```python
from build123d import *

# Parameters (mm, degrees)
SKETCH1_W            = 254
SKETCH1_H            = 203.2
BOSS_EXTRUDE2_DEPTH  = 12.7
SKETCH2_W            = 254
SKETCH2_H            = 203.2
SKETCH2_W_2          = 228.6
SKETCH2_H_2          = 177.8
BOSS_EXTRUDE3_DEPTH  = 12.7
SKETCH6_R            = 6.35
CUT_EXTRUDE2_DEPTH   = 52.07
SKETCH8_R            = 6.35
CUT_EXTRUDE3_DEPTH   = 52.07
SKETCH9_R            = 3.302
BOSS_EXTRUDE5_DEPTH  = 25.4
SKETCH10_R           = 6.35
CUT_EXTRUDE4_DEPTH   = 45.212
SKETCH11_R           = 6.35
CUT_EXTRUDE5_DEPTH   = 190.246
SKETCH12_R           = 5.842
SKETCH12_R_2         = 3.302
BOSS_EXTRUDE6_DEPTH  = 24.13
SKETCH15_R           = 6.35
CUT_EXTRUDE6_DEPTH   = 1.27
SKETCH17_R           = 3.302
BOSS_EXTRUDE7_DEPTH  = 1.27
SKETCH18_R           = 3.302
BOSS_EXTRUDE8_DEPTH  = 1.27
SKETCH19_R           = 5.842
SKETCH19_R_2         = 3.302
BOSS_EXTRUDE9_DEPTH  = 73.025
CUT_EXTRUDE7_DEPTH   = 7.62
SKETCH21_R           = 6.35
BOSS_EXTRUDE10_DEPTH = 12.7
SKETCH23_R           = 6.35
BOSS_EXTRUDE11_DEPTH = 12.7
SKETCH24_R           = 3.81
CUT_EXTRUDE8_DEPTH   = 167.132
FILLET1_R            = 5.08


with BuildPart() as part:
    # Sketch1 → Boss-Extrude2 (new body)
    with BuildSketch(Plane(origin=(0, 0, 0), x_dir=(1, 0, 0), z_dir=(0, 1, 0))):
        with Locations((127, 101.6)):
            Rectangle(SKETCH1_W, SKETCH1_H)
    extrude(amount=BOSS_EXTRUDE2_DEPTH)

    # Sketch2 → Boss-Extrude3 (add)
    with BuildSketch(Plane(origin=(0, 0, 0), x_dir=(-1, 0, 0), z_dir=(0, -1, 0))):
        with Locations((-127, 101.6)):
            Rectangle(SKETCH2_W, SKETCH2_H)
        with Locations((-127, 101.6)):
            Rectangle(SKETCH2_W_2, SKETCH2_H_2, mode=Mode.SUBTRACT)
    extrude(amount=BOSS_EXTRUDE3_DEPTH)

    # Sketch6 → Cut-Extrude2 (cut)
    with BuildSketch(Plane(origin=(228.6, 0, 0), x_dir=(0, 0, -1), z_dir=(1, 0, 0))):
        with Locations((0, -12.7)):
            Circle(SKETCH6_R)
    extrude(amount=-CUT_EXTRUDE2_DEPTH, mode=Mode.SUBTRACT)

    # Sketch8 → Cut-Extrude3 (cut)
    with BuildSketch(Plane.ZY.offset(-25.4)):
        with Locations((0, -12.7)):
            Circle(SKETCH8_R)
    extrude(amount=-CUT_EXTRUDE3_DEPTH, mode=Mode.SUBTRACT)

    # Sketch9 → Boss-Extrude5 (add)
    with BuildSketch(Plane(origin=(228.6, 0, 0), x_dir=(0, 0, -1), z_dir=(1, 0, 0))):
        with BuildLine():
            Line((0, -4.734153711), (0, -6.858))
            ThreePointArc((0, -6.858), (-4.130917816, -16.830917816), (5.842, -12.7))
            Line((5.842, -12.7), (6.842694324, -12.7))
            Line((6.842694324, -12.7), (6.842694324, -8.927228158))
            Line((6.842694324, -8.927228158), (0, -4.734153711))
        make_face()
        with Locations((0, -12.7)):
            Circle(SKETCH9_R, mode=Mode.SUBTRACT)
    extrude(amount=-BOSS_EXTRUDE5_DEPTH)

    # Sketch10 → Cut-Extrude4 (cut)
    with BuildSketch(Plane(origin=(228.6, 0, 0), x_dir=(0, 0, -1), z_dir=(1, 0, 0))):
        with Locations((0, -12.7)):
            Circle(SKETCH10_R)
    extrude(amount=CUT_EXTRUDE4_DEPTH, mode=Mode.SUBTRACT)

    # Sketch11 → Cut-Extrude5 (cut)
    with BuildSketch(Plane(origin=(176.53, 0, 0), x_dir=(0, 0, -1), z_dir=(1, 0, 0))):
        with Locations((0, -12.7)):
            Circle(SKETCH11_R)
    extrude(amount=-CUT_EXTRUDE5_DEPTH, mode=Mode.SUBTRACT)

    # Sketch12 → Boss-Extrude6 (add)
    with BuildSketch(Plane.ZY):
        with BuildLine():
            ThreePointArc((-5.842, -12.7), (-4.130917816, -8.569082184), (0, -6.858))
            Line((0, -6.858), (0, -6.35))
            ThreePointArc((0, -6.35), (-4.490128061, -8.209871939), (-6.35, -12.7))
            Line((-6.35, -12.7), (-5.842, -12.7))
        make_face()
        with Locations((0, -12.7)):
            Circle(SKETCH12_R)
        with Locations((0, -12.7)):
            Circle(SKETCH12_R_2, mode=Mode.SUBTRACT)
    extrude(amount=-BOSS_EXTRUDE6_DEPTH)

    # Sketch15 → Cut-Extrude6 (cut)
    with BuildSketch(Plane(origin=(228.6, 0, 0), x_dir=(0, 0, -1), z_dir=(1, 0, 0))):
        with Locations((0, -12.7)):
            Circle(SKETCH15_R)
    extrude(amount=-CUT_EXTRUDE6_DEPTH, mode=Mode.SUBTRACT)

    # Sketch17 → Boss-Extrude7 (add)
    with BuildSketch(Plane.ZY.offset(-203.2)):
        with BuildLine():
            ThreePointArc((-5.842, -12.7), (-4.130917816, -8.569082184), (0, -6.858))
            Line((0, -6.858), (0, -6.35))
            ThreePointArc((0, -6.35), (-4.490128061, -8.209871939), (-6.35, -12.7))
            Line((-6.35, -12.7), (-5.842, -12.7))
        make_face()
        with BuildLine():
            ThreePointArc((5.842, -12.7), (4.130917816, -8.569082184), (0, -6.858))
            ThreePointArc((0, -6.858), (-4.130917816, -8.569082184), (-5.842, -12.7))
            ThreePointArc((-5.842, -12.7), (0, -18.542), (5.842, -12.7))
        make_face()
        with Locations((0, -12.7)):
            Circle(SKETCH17_R, mode=Mode.SUBTRACT)
    extrude(amount=BOSS_EXTRUDE7_DEPTH)

    # Sketch18 → Boss-Extrude8 (add)
    with BuildSketch(Plane(origin=(24.13, 0, 0), x_dir=(0, 0, -1), z_dir=(1, 0, 0))):
        with BuildLine():
            Line((0, -6.35), (0, -6.858))
            ThreePointArc((0, -6.858), (4.130917816, -8.569082184), (5.842, -12.7))
            Line((5.842, -12.7), (6.35, -12.7))
            ThreePointArc((6.35, -12.7), (4.490128061, -8.209871939), (0, -6.35))
        make_face()
        with BuildLine():
            ThreePointArc((5.842, -12.7), (4.130917816, -8.569082184), (0, -6.858))
            ThreePointArc((0, -6.858), (-4.130917816, -16.830917816), (5.842, -12.7))
        make_face()
        with Locations((0, -12.7)):
            Circle(SKETCH18_R, mode=Mode.SUBTRACT)
    extrude(amount=BOSS_EXTRUDE8_DEPTH)

    # Sketch19 → Boss-Extrude9 (add)
    with BuildSketch(Plane.ZY.offset(-53.34)):
        with BuildLine():
            ThreePointArc((-5.842, -12.7), (-4.130917816, -8.569082184), (0, -6.858))
            Line((0, -6.858), (0, -5.334694101))
            Line((0, -5.334694101), (-5.217733662, -7.625492191))
            Line((-5.217733662, -7.625492191), (-6.523890468, -10.619605484))
            Line((-6.523890468, -10.619605484), (-6.724837669, -12.7))
            Line((-6.724837669, -12.7), (-5.842, -12.7))
        make_face()
        with Locations((0, -12.7)):
            Circle(SKETCH19_R)
        with Locations((0, -12.7)):
            Circle(SKETCH19_R_2, mode=Mode.SUBTRACT)
    extrude(amount=-BOSS_EXTRUDE9_DEPTH)

    # Sketch3 → Cut-Extrude7 (cut)
    with BuildSketch(Plane(origin=(0, 12.7, 0), x_dir=(1, 0, 0), z_dir=(0, 1, 0))):
        with BuildLine():
            Line((195.366950221, 165.545782342), (91.71222682, 165.545782342))
            add(Edge.make_bspline(
                [(91.71222682, 165.545782342), (67.539208551, 163.235170178), (59.846395191, 139.038085668)],
                knots=[0, 0, 0, 1, 1, 1], degree=2))
            Line((59.846395191, 139.038085668), (125.30712104, 139.038085668))
            add(Edge.make_bspline(
                [(125.30712104, 139.038085668), (126.780616205, 139.122377702), (126.96048329, 137.769188416)],
                knots=[0, 0, 0, 1, 1, 1], degree=2))
            Line((126.96048329, 137.769188416), (126.96048329, 132.272484091))
            add(Edge.make_bspline(
                [(126.96048329, 132.272484091), (126.876874172, 130.733531241), (128.303731924, 130.371199046)],
                knots=[0, 0, 0, 1, 1, 1], degree=2))
            Line((128.303731924, 130.371199046), (162.187188306, 130.371199046))
            add(Edge.make_bspline(
                [(195.366950221, 165.545782342), (193.745607246, 135.56730888), (162.187188306, 130.371199046)],
                knots=[0, 0, 0, 1, 1, 1], degree=2))
        make_face()
        with BuildLine():
            Line((161.642347888, 119.295964928), (128.497808789, 119.295964928))
            add(Edge.make_bspline(
                [(128.497808789, 119.295964928), (127.070096751, 118.926569019), (126.96048329, 117.397764841)],
                knots=[0, 0, 0, 1, 1, 1], degree=2))
            Line((126.96048329, 117.397764841), (126.96048329, 112.151116085))
            add(Edge.make_bspline(
                [(126.96048329, 112.151116085), (126.743790117, 110.899444942), (125.464733978, 110.784690654)],
                knots=[0, 0, 0, 1, 1, 1], degree=2))
            Line((125.464733978, 110.784690654), (59.846395191, 110.784690654))
            add(Edge.make_bspline(
                [(59.846395191, 110.784690654), (61.887337052, 98.301496186), (73.317351169, 93.027012339)],
                knots=[0, 0, 0, 1, 1, 1], degree=2))
            Line((73.317351169, 93.027012339), (125.464733978, 93.027012339))
            add(Edge.make_bspline(
                [(125.464733978, 93.027012339), (126.711731964, 92.919963041), (126.96048329, 91.748824412)],
                knots=[0, 0, 0, 1, 1, 1], degree=2))
            Line((126.96048329, 91.748824412), (126.96048329, 85.74475013))
            add(Edge.make_bspline(
                [(126.96048329, 85.74475013), (127.024328685, 84.195885842), (128.497808789, 83.912442397)],
                knots=[0, 0, 0, 1, 1, 1], degree=2))
            Line((128.497808789, 83.912442397), (195.366950221, 83.912442397))
            add(Edge.make_bspline(
                [(161.642347888, 119.295964928), (193.222633695, 115.013388161), (195.366950221, 83.912442397)],
                knots=[0, 0, 0, 1, 1, 1], degree=2))
        make_face()
        with BuildLine():
            Line((195.366950221, 72.802355269), (128.303731924, 72.802355269))
            add(Edge.make_bspline(
                [(128.303731924, 72.802355269), (127.014045367, 72.648063165), (126.96048329, 71.297279055)],
                knots=[0, 0, 0, 1, 1, 1], degree=2))
            Line((126.96048329, 71.297279055), (126.96048329, 66.07466352))
            add(Edge.make_bspline(
                [(126.96048329, 66.07466352), (126.573968469, 64.92692802), (125.30712104, 64.769219048)],
                knots=[0, 0, 0, 1, 1, 1], degree=2))
            Line((125.30712104, 64.769219048), (74.082862231, 64.769219048))
            add(Edge.make_bspline(
                [(74.082862231, 64.769219048), (58.4794695, 55.884745917), (58.811181594, 37.622601841)],
                knots=[0, 0, 0, 1, 1, 1], degree=2))
            Line((58.811181594, 37.622601841), (162.716666362, 37.622601841))
            add(Edge.make_bspline(
                [(162.716666362, 37.622601841), (194.140729717, 41.705995139), (195.366950221, 72.802355269)],
                knots=[0, 0, 0, 1, 1, 1], degree=2))
        make_face()
    extrude(amount=-CUT_EXTRUDE7_DEPTH, mode=Mode.SUBTRACT)

    # Sketch21 → Boss-Extrude10 (add)
    with BuildSketch(Plane(origin=(177.8, 0, 0), x_dir=(0, 0, -1), z_dir=(1, 0, 0))):
        with BuildLine():
            Line((203.2, 6.35), (203.2, 0))
            Line((203.2, 0), (203.2, -6.35))
            Line((203.2, -6.35), (213.36, -6.35))
            ThreePointArc((213.36, -6.35), (207.01, 0), (213.36, 6.35))
            Line((213.36, 6.35), (203.2, 6.35))
        make_face()
        with Locations((213.36, 0)):
            Circle(SKETCH21_R)
    extrude(amount=BOSS_EXTRUDE10_DEPTH)

    # Sketch23 → Boss-Extrude11 (add)
    with BuildSketch(Plane(origin=(76.2, 0, 0), x_dir=(0, 0, -1), z_dir=(1, 0, 0))):
        with BuildLine():
            Line((213.36, 6.35), (203.2, 6.35))
            Line((203.2, 6.35), (203.2, -6.35))
            Line((203.2, -6.35), (213.36, -6.35))
            ThreePointArc((213.36, -6.35), (207.01, 0), (213.36, 6.35))
        make_face()
        with Locations((213.36, 0)):
            Circle(SKETCH23_R)
    extrude(amount=-BOSS_EXTRUDE11_DEPTH)

    # Sketch24 → Cut-Extrude8 (cut)
    with BuildSketch(Plane.ZY.offset(-63.5)):
        with Locations((-213.36, 0)):
            Circle(SKETCH24_R)
    extrude(amount=-CUT_EXTRUDE8_DEPTH, mode=Mode.SUBTRACT)

    # Fillet1
    fillet1_edges = [part.edges().sort_by_distance(p)[0] for p in [
        (184.15, -6.35, -203.2),
        (184.15, 6.35, -203.2),
        (69.85, -6.35, -203.2),
        (69.85, 6.35, -203.2),
    ]]
    fillet(fillet1_edges, radius=FILLET1_R)


solid = part.part
```
Input: part model. Units: mm. Frame: model coordinates. A direction names the side the tool comes from. Give positions to 0.01 mm unless a question says otherwise; leave off trailing zeros. Order: outer loops, then holes, each group sorted by start corner. A loop starts at its lowest first (then second) coordinate and runs counter-clockwise, first axis right, second up.
1. Cut plane B-B (x = 69.5). State how many separate pieces and enclosed holes the cut face has, and give its area (3 significant figures).
Computed:
separate pieces: 1
enclosed holes: 2
area: 2,680 mm2
2. Line query: probe 1 along X at (y, z) = (-6.5, -50); probe 2 along Y at (x, z) = (182, -213); probe 3 along X at (y, z) = (-11.5, -5) (3 decimals). Output: solid intervals per line, ascending.
Computed:
probe 1: x = 0 to 12.7, 241.3 to 254
probe 2: y = -6.35 to -3.79, 3.79 to 6.35
probe 3: x = 0 to 25.4, 53.34 to 126.365, 201.93 to 227.33
3. Pin query (flat end, axial travel): pin 1 Ø7 at (y, z) = (0, -213.36) entering from -X; pin 2 Ø1 at (x, y) = (57, -14) entering from -Z; pin 3 Ø3.5 at (y, z) = (-10.5, 3) entering from +X; pin 4 Ø2.5 at (x, y) = (167, 9) entering from +Z. Return the tip coordinate at first contact, or that it passes through.
Computed:
pin 1: passes through
pin 2: stops at z = -5.79
pin 3: stops at x = 227.33
pin 4: stops at z = 0
4. Draft query along Z for faces 1 (the face through (184.06, -0.14, -219.71)), 2 (the face through (145, 9, -119.296)), 3 (the face through (25.4, -15, -3)). Return one class per face: released by +Z, released by -Z, zero draft, split by the parting line, or undercut.
Computed:
face 1: released by -Z
face 2: undercut
face 3: zero draft
5. Cut plane A-A (x = 97.5). Return loops of the section in (y, z), and give its area (3 significant figures).
Computed:
outline: (-12.7, -203.2) - (12.7, -203.2) - (12.7, -165.55) - (5.08, -165.55) - (5.08, -139.04) - (12.7, -139.04) - (12.7, -110.78) - (5.08, -110.78) - (5.08, -93.03) - (12.7, -93.03) - (12.7, -64.77) - (5.08, -64.77) - (5.08, -37.62) - (12.7, -37.62) - (12.7, 0) - (-6.86, 0) arc R5.84 ccw (long way) to (-12.7, -5.84) - (-12.7, -12.7) - (0, -12.7) - (0, -190.5) - (-12.7, -190.5) - close; hole circle Ø6.6 at (-12.7, 0)
area: 2,410 mm2
6. Set-up query: faces 4 (the face through (126.96, 9, -69)), 5 (the face through (126.365, -9.65, -1.69)), 6 (the face through (227.33, -15, -3)), 7 (the face through (125, 0, -103)). Return all of +Z, -Z, +X, -X, +Y, -Y with unobstructed straight access to the full face (end or side cutting, diameter ignored); none if empty.
Computed:
face 4: +Y
face 5: +Z, -Y
face 6: +Z, +X, -Y
face 7: -Y
